Model file for the job. Use its own axes, mm. Round coordinates to 2 decimals unless told otherwise and drop trailing zeros. Write each loop counter-clockwise with the first axis right and the second up, starting at its lowest first coordinate (ties: lowest second). Pieces come first, ordered by that corner, then holes. Notation, with made-up numbers: (-23.5, 75.25) - (20.5, 75.25) arc R20 cw to (20.5, 96.25) - close; hole circle Ø8 at (68.25, 31). An arc over 180 degrees is marked (long way). One line per item, written item: value.
from build123d import *
from OCP.BRepFilletAPI import BRepFilletAPI_MakeChamfer

# Parameters (mm, degrees)
SKETCH1_W           = 70
SKETCH1_H           = 20
BOSS_EXTRUDE1_DEPTH = 20
CHAMFER1_SIZE       = 17
CHAMFER1_SIZE2      = 5


with BuildPart() as part:
    # Sketch1 → Boss-Extrude1 (new body)
    with BuildSketch(Plane(origin=(0, 0, 0), x_dir=(1, 0, 0), z_dir=(0, 1, 0))):
        with Locations((35, 10)):
            Rectangle(SKETCH1_W, SKETCH1_H)
    extrude(amount=BOSS_EXTRUDE1_DEPTH)

    # Chamfer1: one chamfer whose edges measure the first distance from different faces: ONE call of the kernel's chamfer builder (chamfer() names one face for all edges)
    chamfer1_edges_1 = [part.edges().sort_by_distance(p)[0] for p in [
        (35, 20, -20),
    ]]
    chamfer1_side_1 = [part.faces().sort_by_distance(p)[0] for p in [
        (35, 10, -20),
    ]]
    chamfer1_edges_2 = [part.edges().sort_by_distance(p)[0] for p in [
        (35, 20, 0),
    ]]
    chamfer1_side_2 = [part.faces().sort_by_distance(p)[0] for p in [
        (35, 10, 0),
    ]]
    chamfer1 = BRepFilletAPI_MakeChamfer(part.part.solid().wrapped)
    for e in chamfer1_edges_1:
        chamfer1.Add(CHAMFER1_SIZE, CHAMFER1_SIZE2, e.wrapped, chamfer1_side_1[0].wrapped)  # the first distance lies on this face
    for e in chamfer1_edges_2:
        chamfer1.Add(CHAMFER1_SIZE, CHAMFER1_SIZE2, e.wrapped, chamfer1_side_2[0].wrapped)  # the first distance lies on this face
    add(Compound.cast(chamfer1.Shape()), mode=Mode.REPLACE)


solid = part.part
1. Band-saw the part on B-B on z = -4.25. Write the cut outline in (x, y), plus the area to 3 significant figures.
Report:
outline: (0, 0) - (70, 0) - (70, 17.45) - (0, 17.45) - close
area: 1,220 mm²
2. Band-saw the part on C-C on y = 18. Write the cut outline in (x, z).
Report:
outline: (0, -15.59) - (70, -15.59) - (70, -4.41) - (0, -4.41) - close
3. Band-saw the part on A-A on x = 11. Write the cut outline in (y, z).
Report:
outline: (0, -20) - (3, -20) - (20, -15) - (20, -5) - (3, 0) - (0, 0) - close
4. Drop flat-ended pins along their axis: pin 1 (12 mm diameter, centred on x = 9.5, y = 9.5, fed in from +Z); pin 2 (2 mm diameter, centred on x = 12.5, y = 17, fed in from +Z). Give the stop position or say it passes through.
Report:
pin 1: z = -0.15
pin 2: z = -3.82
5. Wall check: probe 1 along Z at (x, y) = (28.5, 5); probe 2 along Z at (x, y) = (46, 17.5). Give the ranges that are in metal, low to high. Write a range as [from, to].
Report:
probe 1: [-19.41, -0.59]
probe 2: [-15.74, -4.26]
